Geometry: see drawing. Coordinates: mm, zero at the bounding-box minimum. Give positions to 0.01 mm unless a question says otherwise; leave off trailing zeros. Loops run counter-clockwise (first coordinate to the right, second up) from the corner with the lowest first, then second, coordinate; pieces in that order, holes last. Notation, with made-up numbers: M -8,29 L 25,29 A12 cw 25,44 Z; hole C 19.25,22 d1. An arc over 180 degrees is marked long. Put each result on its own line as item: value.
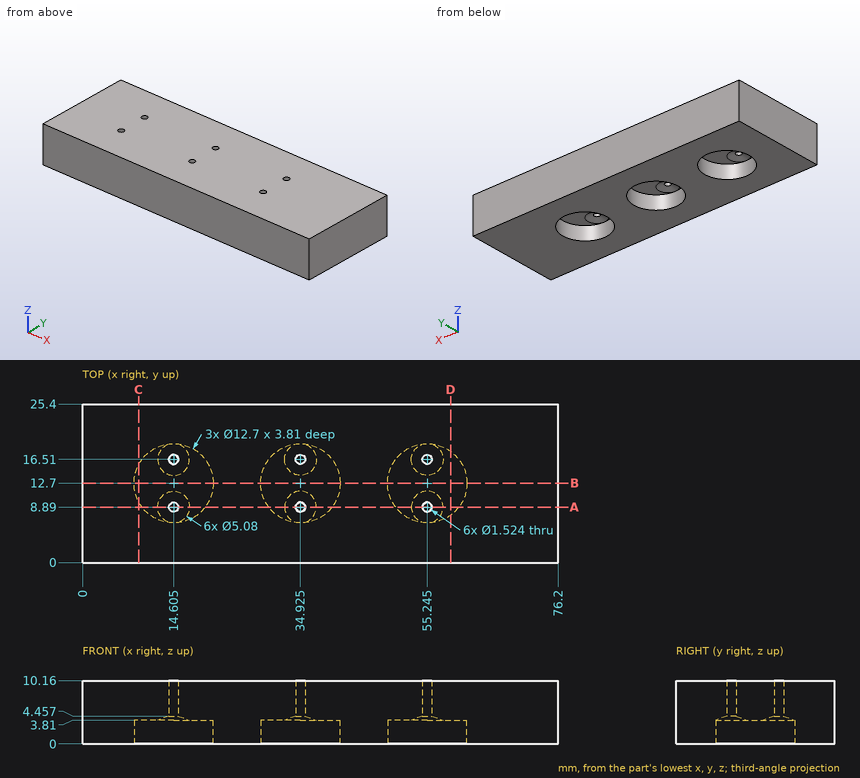
Item 1: Section C-C on x = 9. Output: boundary loops of the cut face in (y, z), then the cut area to 3 significant figures.
Output values:
outline: M 0,0 L 9.72,0 L 9.72,3.81 L 15.68,3.81 L 15.68,0 L 25.4,0 L 25.4,10.16 L 0,10.16 Z
area: 235 mm²
Item 2: Section D-D on x = 59. Output: boundary loops of the cut face in (y, z).
Output values:
outline: M 0,0 L 7.58,0 L 7.58,3.81 L 17.82,3.81 L 17.82,0 L 25.4,0 L 25.4,10.16 L 0,10.16 Z
Item 3: Pin query (flat end, axial travel): pin 1 Ø7.5 at (x, y) = (34.925, 12.7) entering from -Z; pin 2 Ø2.5 at (x, y) = (14.605, 16.51) entering from -Z; pin 3 Ø1.8 at (x, y) = (55.245, 16.51) entering from -Z. Return the tip coordinate at first contact, or that it passes through.
Output values:
pin 1: z = 3.81
pin 2: z = 4.28
pin 3: z = 4.41
Item 4: Line query: probe 1 along X at (y, z) = (16.51, 8.8); probe 2 along X at (y, z) = (8.5, 3); probe 3 along Y at (x, z) = (15.5, 0.5). Output: solid intervals per line, ascending. Write a range as [from, to].
Output values:
probe 1: [0, 13.84], [15.37, 34.16], [35.69, 54.48], [56.01, 76.2]
probe 2: [0, 9.84], [19.37, 30.16], [39.69, 50.48], [60.01, 76.2]
probe 3: [0, 6.41], [18.99, 25.4]
Item 5: Section B-B on y = 12.7. Output: boundary loops of the cut face in (x, z) (3 decimals), then the cut area to 3 significant figures.
Output values:
outline: M 0,0 L 8.255,0 L 8.255,3.81 L 20.955,3.81 L 20.955,0 L 28.575,0 L 28.575,3.81 L 41.275,3.81 L 41.275,0 L 48.895,0 L 48.895,3.81 L 61.595,3.81 L 61.595,0 L 76.2,0 L 76.2,10.16 L 0,10.16 Z
area: 629 mm²
Item 6: Section A-A on y = 8.89. Count the separate pieces of the cut face and the enclosed holes in it, then the cut area to 3 significant figures.
Output values:
separate pieces: 4
enclosed holes: 0
area: 626 mm²
